Drawing for the job (mm, zero at the part's lowest x, y, z). Coordinates: 2 decimals unless noted, no trailing zeros. Order: outer loops, then holes, each group sorted by start corner. A loop starts at its lowest first (then second) coordinate and runs counter-clockwise, first axis right, second up. Notation, with made-up numbers: M 47.5,-15 L 101.5,-15 A29 cw 101.5,10 Z; hole C -8,-0.5 d6. An arc over 180 degrees is marked long. Write item = value, one per line. Start each with the question number.
Q1. Drill centre lines: probe 1 along Y at (x, z) = (2, 3.3) (1 decimal); probe 2 along Y at (x, z) = (2.25, 3.05) (1 decimal); probe 3 along X at (y, z) = (3, 1.75). Where is each one in solid material? Low to high.
Q2. Pin check, flat tip, straight feed: P1, Ø1, axis at x = 5, z = 1, coming from the -Y side. Stop position of the tip, or through.
Q3. Pull direction X, two halves, no side cores. Call the marked faces 1, 2 and 3: released by +X, released by -X, zero draft, split by the parting line, or undercut.
Q4. Band-saw the part on A-A on y = 2.75. Write the cut outline in (x, z).
Q5. Band-saw the part on C-C on z = 2.5. Write the cut outline in (x, y) (1 decimal), plus the area to 3 significant figures.
Q6. Band-saw the part on B-B on x = 2. Write the cut outline in (y, z) (1 decimal).
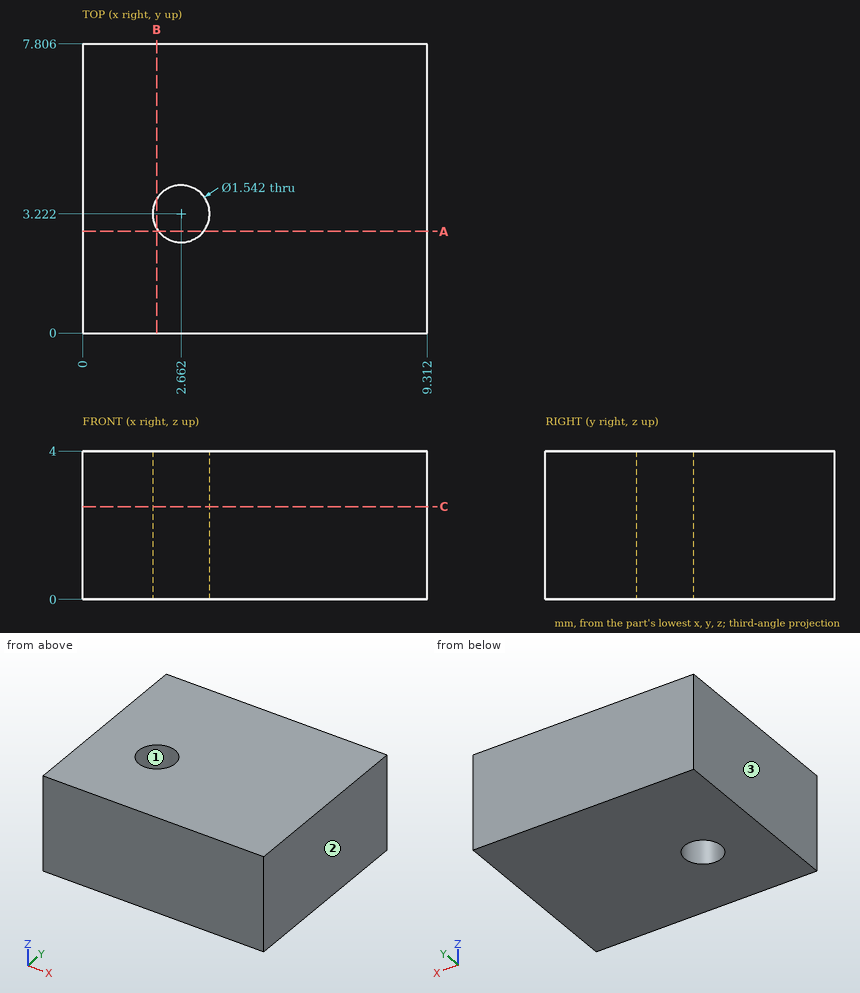
Recorded:
q1.probe_1 = 0 to 2.8, 3.6 to 7.8
q1.probe_2 = 0 to 2.6, 3.9 to 7.8
q1.probe_3 = 0 to 1.92, 3.4 to 9.31
q2.P1 = 0
q3.face_1 = undercut
q3.face_2 = released by +X
q3.face_3 = released by -X
q4.outline = M 0,0 L 2.05,0 L 2.05,4 L 0,4 Z; M 3.27,0 L 9.31,0 L 9.31,4 L 3.27,4 Z
q5.outline = M 0,0 L 9.3,0 L 9.3,7.8 L 0,7.8 Z; hole C 2.7,3.2 d1.5
q5.area = 70.8 mm2
q6.outline = M 0,0 L 2.8,0 L 2.8,4 L 0,4 Z; M 3.6,0 L 7.8,0 L 7.8,4 L 3.6,4 Z
